Model file for the job. Use its own axes, mm. Face numbers are marked on the shaded views. A direction names the side the tool comes from. Coordinates: 2 decimals unless noted, no trailing zeros. Write each loop counter-clockwise with the first axis right and the second up, starting at its lowest first coordinate (ties: lowest second). Pieces come first, ordered by that corner, then holes. Notation, with made-up numbers: M 46,-34.5 L 88,-34.5 A23 cw 88,-7.5 Z; hole C -38.75,1.5 d5. An arc over 180 degrees is marked long. Put each result on its own line as item: value. Start each with the question number.
Q1. Which spindle directions (+Z, -Z, +X, -X, +Y, -Y) get a long thin tool onto all of the face, cutting with end or side? Do the marked faces 1, 2 and 3. Say none if no direction does.
Q2. Drop flat-ended pins along their axis: pin 1 (1.5 mm diameter, centred on x = -32, z = -17, fed in from +Y); pin 2 (9.5 mm diameter, centred on x = 4.5, y = -37, fed in from -Z); pin 3 (1.9 mm diameter, centred on x = 35.75, y = -20.64, fed in from +Z); pin 4 (1 mm diameter, centred on x = 1, z = -1, fed in from -Y). Give the stop position or say it passes through.
Q3. Cut at A-A (y = 0). Write the cut outline in (x, z), then the cut area to 3 significant figures.
Q4. Pull direction Y, two halves, no side cores. Call the marked faces 4, 5, 6 and 7: pulls with the +Y half, pulls with the -Y half, needs draft (parallel to the pull), parting line crosses it, or undercut.
Q5. Drill centre lines: line 1 along X through (y, z) = (-50, 4); line 2 along Z through (x, y) = (-39, 1); line 3 along X through (y, z) = (-68, -3). Where is each one in solid material? Low to high.
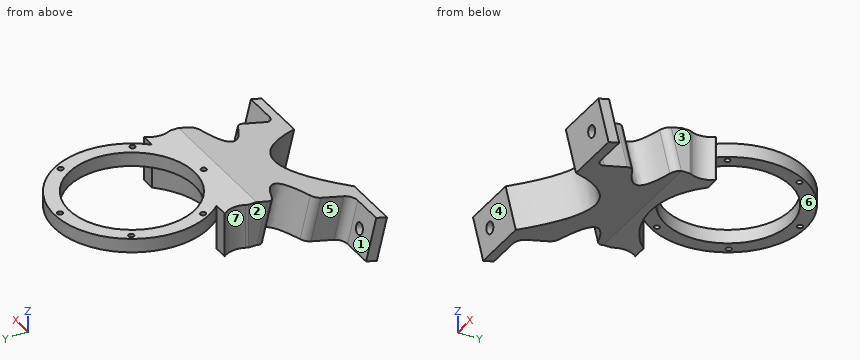
```python
from build123d import *
from build123d.topology import SkipClean

# Parameters (mm, degrees)
SKETCH1_R                       = 44.45
SKETCH1_R_2                     = 36.0426
SKETCH1_R_3                     = 1.575
BOSS_EXTRUDE1_DEPTH             = 8
BOSS_EXTRUDE2_START             = -25.4
BOSS_EXTRUDE2_DEPTH             = 25.4
SKETCH5_W                       = 127
SKETCH5_H                       = 24.677347648
BOSS_EXTRUDE3_DEPTH             = 22.86
BOSS_EXTRUDE3_DIRECTION_2_REACH = 117.98
CUT_EXTRUDE1_DEPTH              = 103.517532245
CUT_EXTRUDE2_DEPTH              = 106.121352295
SKETCH8_R                       = 3.2639
CUT_EXTRUDE3_DEPTH              = 132.797554186
SKETCH10_W                      = 23.84426271
SKETCH10_H                      = 24.677347648
SKETCH10_R                      = 3.2639
BOSS_EXTRUDE4_DEPTH             = 34.23412
FILLET3_START                   = -19.427790223
FILLET3_DEPTH                   = 24.677347648
FILLET4_R                       = 12.7
SKETCH11_W                      = 23.84426271
SKETCH11_H                      = 32.29864
CUT_EXTRUDE4_DEPTH              = 134.162391299
BOSS_EXTRUDE5_DEPTH             = 24.677347648
FILLET5_R                       = 5.08
CUT_EXTRUDE5_DEPTH              = 134.162391299
CUT_EXTRUDE6_DEPTH              = 134.162391464
FILLET6_START                   = -20
FILLET6_DEPTH                   = 26.377499095


with BuildPart() as part:
    # Sketch1 → Boss-Extrude1 (new body)
    with BuildSketch(Plane.XY):
        Circle(SKETCH1_R)
        Circle(SKETCH1_R_2, mode=Mode.SUBTRACT)
        with Locations((35.745198541, 20.6375)):
            Circle(SKETCH1_R_3, mode=Mode.SUBTRACT)
        with Locations((0, 41.275)):
            Circle(SKETCH1_R_3, mode=Mode.SUBTRACT)
        with Locations((-35.745198541, 20.6375)):
            Circle(SKETCH1_R_3, mode=Mode.SUBTRACT)
        with Locations((-35.745198541, -20.6375)):
            Circle(SKETCH1_R_3, mode=Mode.SUBTRACT)
        with Locations((0, -41.275)):
            Circle(SKETCH1_R_3, mode=Mode.SUBTRACT)
        with Locations((35.745198541, -20.6375)):
            Circle(SKETCH1_R_3, mode=Mode.SUBTRACT)
    extrude(amount=BOSS_EXTRUDE1_DEPTH)

    # Sketch4 → Boss-Extrude2 (add)
    with BuildSketch(Plane.XY.offset(8).offset(BOSS_EXTRUDE2_START)):
        with BuildLine():
            Line((-39.65573729, -44.45), (-63.5, -44.45))
            Line((-63.5, -44.45), (-63.5, -49.2125))
            Line((-63.5, -49.2125), (63.5, -49.2125))
            Line((63.5, -49.2125), (63.5, -44.45))
            Line((63.5, -44.45), (39.65573729, -44.45))
            Line((39.65573729, -44.45), (36.050670263, -35.790909091))
            ThreePointArc((36.050670263, -35.790909091), (38.587710733, -33.039802972), (40.915335308, -30.10938951))
            Line((40.915335308, -30.10938951), (32.699039181, -30.10938951))
            ThreePointArc((32.699039181, -30.10938951), (0, -44.45), (-32.699039181, -30.10938951))
            Line((-32.699039181, -30.10938951), (-40.915335308, -30.10938951))
            ThreePointArc((-40.915335308, -30.10938951), (-38.587710733, -33.039802972), (-36.050670263, -35.790909091))
            Line((-36.050670263, -35.790909091), (-39.65573729, -44.45))
        make_face()
    extrude(amount=BOSS_EXTRUDE2_DEPTH)

    # Sketch5 → Boss-Extrude3 (add)
    with BuildSketch(Plane(origin=(0, -50.455795448, -12.299797104), x_dir=(-1, 0, 0), z_dir=(0, -0.971549119997646, -0.2368381460656192))):
        with Locations((0, -7.089116399)):
            Rectangle(SKETCH5_W, SKETCH5_H)
    extrude(amount=BOSS_EXTRUDE3_DEPTH)

    # Boss-Extrude3 direction 2: up to this face of the body (flat: up to its plane)
    boss_extrude3_direction_2_end = Plane(part.part.faces().sort_by_distance((0, -49.2125, -4.7))[0])
    # Sketch5 → Boss-Extrude3 direction 2 (add, up to the picked face)
    with BuildSketch(Plane(origin=(0, -50.455795448, -12.299797104), x_dir=(-1, 0, 0), z_dir=(0, -0.971549119997646, -0.2368381460656192)), mode=Mode.PRIVATE) as boss_extrude3_direction_2_sk1:
        with Locations((0, -7.089116399)):
            Rectangle(SKETCH5_W, SKETCH5_H)
    boss_extrude3_direction_2_tool1 = split(extrude(boss_extrude3_direction_2_sk1.sketch, amount=-BOSS_EXTRUDE3_DIRECTION_2_REACH, mode=Mode.PRIVATE), bisect_by=boss_extrude3_direction_2_end, keep=Keep.BOTH, mode=Mode.PRIVATE)
    add(boss_extrude3_direction_2_tool1.solids().sort_by(Axis((0, -52.134769, -5.412372), (0, 0.971549119997646, 0.2368381460656192)))[0])

    # Sketch6 → Cut-Extrude1 (cut, through all)
    with BuildSketch(Plane(origin=(0, 1.243295448, -5.100202896), x_dir=(-1, 0, 0), z_dir=(0, 0.23683814606561915, -0.971549119997646))):
        with BuildLine():
            Line((-39.65573729, -74.793344809), (-39.65573729, -84.912644386))
            Line((-39.65573729, -84.912644386), (39.65573729, -84.912644386))
            Line((39.65573729, -84.912644386), (39.65573729, -74.793344809))
            add(Edge.make_bspline(
                [(-39.65573729, -74.793344809), (0, -52.373165884), (39.65573729, -74.793344809)],
                knots=[0, 0, 0, 1, 1, 1], degree=2))
        make_face()
    extrude(amount=-CUT_EXTRUDE1_DEPTH, mode=Mode.SUBTRACT)

    # Sketch7 → Cut-Extrude2 (cut, through all)
    with BuildSketch(Plane(origin=(0, -4.601241819, 18.875052495), x_dir=(1, 0, 0), z_dir=(0, -0.23683814606561915, 0.971549119997646))):
        Polygon((-39.65573729, -41.290653215), (-39.65573729, -70.378824809), (-63.5, -70.378824809), (-63.5, -38.21123826), (-39.65573729, -38.21123826), align=None)
        Polygon((39.65573729, -70.378824809), (63.5, -70.378824809), (63.5, -38.21123826), (39.65573729, -38.21123826), (39.65573729, -41.290653215), align=None)
    extrude(amount=-CUT_EXTRUDE2_DEPTH, mode=Mode.SUBTRACT)

    # Sketch8 → Cut-Extrude3 (cut, through all)
    with BuildSketch(Plane(origin=(0, -68.37648531, -16.66839039), x_dir=(1, 0, 0), z_dir=(0, 0.971549119997646, 0.2368381460656191))):
        with Locations(Location((51.577868645, -7.089116399, 0), (0, 0, 270))):
            Circle(SKETCH8_R)
        with Locations(Location((-51.577868645, -7.089116399, 0), (0, 0, 270))):
            Circle(SKETCH8_R)
    extrude(amount=-CUT_EXTRUDE3_DEPTH, mode=Mode.SUBTRACT)

    # Sketch10 → Boss-Extrude4 (add)
    # profile 1 of 2: a face of its own
    with SkipClean():  # the faces are left unmerged after this step: merging them gives an invalid solid
        with BuildSketch(Plane(origin=(0, -72.665408331, -17.713917123), x_dir=(1, 0, 0), z_dir=(0, -0.9715491199976461, -0.23683814606561926))):
            with Locations((-51.577868645, 7.089116399)):
                Rectangle(SKETCH10_W, SKETCH10_H)
            with Locations(Location((-51.577868645, 7.089116399, 0), (0, 0, 270))):
                Circle(SKETCH10_R, mode=Mode.SUBTRACT)
        # profile 2 of 2: a face of its own
        with BuildSketch(Plane(origin=(0, -72.665408331, -17.713917123), x_dir=(1, 0, 0), z_dir=(0, -0.9715491199976461, -0.23683814606561926))):
            with Locations((51.577868645, 7.089116399)):
                Rectangle(SKETCH10_W, SKETCH10_H)
            with Locations(Location((51.577868645, 7.089116399, 0), (0, 0, 90))):
                Circle(SKETCH10_R, mode=Mode.SUBTRACT)
        extrude(amount=BOSS_EXTRUDE4_DEPTH)
    add(part.part.scale(1), mode=Mode.REPLACE)  # the faces are merged on a copy

    # Fillet3: read off the stored shape, not the designer's step
    # Fillet3 outline → Fillet3 (add)
    with SkipClean():  # the faces are left unmerged after this step: merging them gives an invalid solid
        with BuildSketch(Plane(origin=(0, 0, 0), x_dir=(1, 0, 0), z_dir=(0, 0.23683814606561904, -0.9715491199976461)).offset(FILLET3_START)):
            with BuildLine():
                ThreePointArc((0, 75.867019335), (-23.207224812, 88.40595558), (-39.65573729, 109.027464809))
                Line((-39.65573729, 109.027464809), (-39.65573729, 74.793344809))
                add(Edge.make_bspline(
                    [(39.65573729, 74.793344809), (0, 52.373165884), (-39.65573729, 74.793344809)],
                    knots=[0, 0, 0, 1, 1, 1], degree=2))
                Line((39.65573729, 74.793344809), (39.65573729, 109.027464809))
                ThreePointArc((39.65573729, 109.027464809), (23.207224812, 88.40595558), (0, 75.867019335))
            make_face()
        extrude(amount=FILLET3_DEPTH)

    # Fillet4
    fillet4_edges = [part.edges().sort_by_distance(p)[0] for p in [
        (36.050670263, -35.790909091, -4.7),
        (-36.050670263, -35.790909091, -4.7),
    ]]
    fillet(fillet4_edges, radius=FILLET4_R)

    # Sketch11 → Cut-Extrude4 (cut, through all)
    with BuildSketch(Plane(origin=(0, -4.601241819, 18.875052495), x_dir=(1, 0, 0), z_dir=(0, -0.2368381460656192, 0.9715491199976461))):
        with Locations((-51.577868645, -86.528144809)):
            Rectangle(SKETCH11_W, SKETCH11_H)
        with Locations((51.577868645, -86.528144809)):
            Rectangle(SKETCH11_W, SKETCH11_H)
    extrude(amount=-CUT_EXTRUDE4_DEPTH, mode=Mode.SUBTRACT)

    # Sketch12 → Boss-Extrude5 (add)
    with BuildSketch(Plane(origin=(0, -4.601241819, 18.875052495), x_dir=(1, 0, 0), z_dir=(0, -0.2368381460656192, 0.9715491199976461))):
        Polygon((-39.65573729, -109.027464809), (39.65573729, -109.027464809), (30.485915065, -74.825591671), (-33.624171028, -74.825591671), align=None)
    extrude(amount=-BOSS_EXTRUDE5_DEPTH)

    # Fillet5
    fillet5_edges = [part.edges().sort_by_distance(p)[0] for p in [
        (-39.65573729, -101.435173764, -17.430515609),
        (39.65573729, -101.435173764, -17.430515609),
    ]]
    fillet(fillet5_edges, radius=FILLET5_R)

    # Sketch13 → Cut-Extrude5 (cut, through all)
    with BuildSketch(Plane(origin=(0, -4.601241819, 18.875052495), x_dir=(1, 0, 0), z_dir=(0, -0.2368381460656192, 0.9715491199976461))):
        with BuildLine():
            Line((-30.48, -109.027464809), (-30.48, -117.81515038))
            Line((-30.48, -117.81515038), (30.48, -117.81515038))
            Line((30.48, -117.81515038), (30.48, -109.027464809))
            add(Edge.make_bspline(
                [(-30.48, -109.027464809), (0, -50.4868087), (30.48, -109.027464809)],
                knots=[0, 0, 0, 1, 1, 1], degree=2))
        make_face()
    extrude(amount=-CUT_EXTRUDE5_DEPTH, mode=Mode.SUBTRACT)

    # Sketch14 → Cut-Extrude6 (cut, through all)
    with BuildSketch(Plane(origin=(0, -4.601241819, 18.875052495), x_dir=(1, 0, 0), z_dir=(0, -0.2368381460656192, 0.9715491199976461))):
        with BuildLine():
            Line((-39.65573729, -55.771894755), (-39.65573729, -80.653781316))
            add(Edge.make_bspline(
                [(-39.65573729, -55.771894755), (-5.12128529, -66.290498293), (-39.65573729, -80.653781316)],
                knots=[0, 0, 0, 1, 1, 1], degree=2))
        make_face()
        with BuildLine():
            Line((39.65573729, -80.653781316), (39.65573729, -55.771894755))
            add(Edge.make_bspline(
                [(39.65573729, -55.771894755), (5.12128529, -66.290498293), (39.65573729, -80.653781316)],
                knots=[0, 0, 0, 1, 1, 1], degree=2))
        make_face()
    extrude(amount=-CUT_EXTRUDE6_DEPTH, mode=Mode.SUBTRACT)

    # Fillet6: read off the stored shape, not the designer's step
    # Fillet6 outline → Fillet6 (cut)
    with BuildSketch(Plane(origin=(0, 0, 0), x_dir=(1, 0, 0), z_dir=(0, 0.23683814606561904, -0.9715491199976461)).offset(FILLET6_START)):
        with BuildLine():
            Line((-39.65573729, 55.771894755), (-39.65573729, 52.0803589))
            ThreePointArc((-39.65573729, 52.0803589), (-38.714392857, 55.026191566), (-36.239229378, 56.880274949))
            add(Edge.make_bspline(
                [(-36.239229378, 56.880274949), (-37.853422524, 56.320849013), (-39.65573729, 55.771894755)],
                knots=[0.947811109, 0.947811109, 0.947811109, 1, 1, 1], degree=2))
        make_face()
        with BuildLine():
            add(Edge.make_bspline(
                [(-39.65573729, 80.653781316), (-38.090633643, 80.00283638), (-36.667391198, 79.359788064)],
                knots=[0, 0, 0, 0.045320066, 0.045320066, 0.045320066], degree=2))
            ThreePointArc((-36.667391198, 79.359788064), (-38.843758017, 81.234124448), (-39.65573729, 83.989192337))
            Line((-39.65573729, 83.989192337), (-39.65573729, 80.653781316))
        make_face()
        with BuildLine():
            add(Edge.make_bspline(
                [(39.65573729, 55.771894755), (37.853422524, 56.320849013), (36.239229378, 56.880274949)],
                knots=[0, 0, 0, 0.052188891, 0.052188891, 0.052188891], degree=2))
            ThreePointArc((36.239229378, 56.880274949), (38.714392857, 55.026191566), (39.65573729, 52.0803589))
            Line((39.65573729, 52.0803589), (39.65573729, 55.771894755))
        make_face()
        with BuildLine():
            ThreePointArc((39.65573729, 83.989192337), (38.843758017, 81.234124448), (36.667391198, 79.359788064))
            add(Edge.make_bspline(
                [(36.667391198, 79.359788064), (38.090633643, 80.00283638), (39.65573729, 80.653781316)],
                knots=[0.954679934, 0.954679934, 0.954679934, 1, 1, 1], degree=2))
            Line((39.65573729, 80.653781316), (39.65573729, 83.989192337))
        make_face()
    extrude(amount=FILLET6_DEPTH, mode=Mode.SUBTRACT)


solid = part.part
```
Computed values:
1. face 1: +Z, -X, +Y
1. face 2: +Z, -Z, -X
1. face 3: +Z, -Z, +X
2. pin 1: y = -30.11
2. pin 2: z = 0
2. pin 3: through
2. pin 4: y = -82.01
3. outline: M -44.45,0 L -36.04,0 L -36.04,8 L -44.45,8 Z; M 36.04,0 L 44.45,0 L 44.45,8 L 36.04,8 Z
3. area: 135 mm2
4. face 4: pulls with the -Y half
4. face 5: undercut
4. face 6: needs draft
4. face 7: undercut
5. line 1: -39.66 to 39.66
5. line 2: 0 to 8
5. line 3: -22.41 to 22.41
